CAD build for the part. Positions are in the model's coordinates, mm. A direction names the side the tool comes from. Give positions to 0.01 mm unless a question says otherwise; leave off trailing zeros. Order: outer loops, then holes, each group sorted by start corner. A loop starts at its lowest first (then second) coordinate and runs counter-clockwise, first axis right, second up.
Item 1: Wall check: L1, parallel to Y at x = 105, z = 1.8; L2, parallel to Y at x = 94.5, z = 2.8; L3, parallel to X at y = 18.5, z = 1.75. Give the ranges that are in metal, low to high.
Item 2: Flat gauge pin, fed straight in: P1, Ø2.5, axis at x = 10, y = 10, coming from the +Z side (3 decimals). Where does the tip first touch, or does it go through?
Item 3: Band-saw the part on A-A on y = 18. Give the cut face in (x, z).
Item 4: Two-plate mould, pull along X, no slides. Class faces 1 (the flat face through (56, 18, 0)), 2 (the cylindrical face through (10.761, 8.536, 1.479)), 3 (the flat face through (113, 18, 1)): released by +X, released by -X, zero draft, split by the parting line, or undercut.
Item 5: Band-saw the part on B-B on x = 18. Give the cut face in (y, z).
Item 6: Band-saw the part on D-D on x = 67.5. Give the cut face in (y, z).
Item 7: Which spindle directions (+Z, -Z, +X, -X, +Y, -Y) get a long thin tool onto all of the face, cutting with end or side? Do faces 4 (the cylindrical face through (0.57, 0.6, 1.52)), 5 (the cylindrical face through (24.35, 25.96, 1.48)). Say none if no direction does.
Item 8: Band-saw the part on C-C on z = 1.5. Count the separate pieces of the cut face and the enclosed holes in it, plus the area to 3 significant figures.
```python
from build123d import *

# Parameters (mm, degrees)
SKETCH_1_W      = 113
SKETCH_1_H      = 36
SKETCH_1_R      = 1.65
EXTRUDE_1_DEPTH = 3
FILLET_1_R      = 2


with BuildPart() as part:
    # 草图1 → 凸台-拉伸1 (new body)
    with BuildSketch(Plane.XY):
        with Locations((56.5, 18)):
            Rectangle(SKETCH_1_W, SKETCH_1_H)
        with Locations((10, 10)):
            Circle(SKETCH_1_R, mode=Mode.SUBTRACT)
        with Locations((18, 10)):
            Circle(SKETCH_1_R, mode=Mode.SUBTRACT)
        with BuildLine():
            ThreePointArc((26, 8.35), (24.35, 10), (26, 11.65))
            Line((26, 11.65), (97, 11.65))
            ThreePointArc((97, 11.65), (98.166726189, 11.166726189), (98.65, 10))
            ThreePointArc((98.65, 10), (98.166726189, 8.833273811), (97, 8.35))
            Line((97, 8.35), (26, 8.35))
        make_face(mode=Mode.SUBTRACT)
        with Locations((105, 10)):
            Circle(SKETCH_1_R, mode=Mode.SUBTRACT)
        with Locations((10, 18)):
            Circle(SKETCH_1_R, mode=Mode.SUBTRACT)
        with Locations((18, 18)):
            Circle(SKETCH_1_R, mode=Mode.SUBTRACT)
        with Locations((10, 26)):
            Circle(SKETCH_1_R, mode=Mode.SUBTRACT)
        with Locations((18, 26)):
            Circle(SKETCH_1_R, mode=Mode.SUBTRACT)
        with BuildLine():
            ThreePointArc((26, 24.35), (24.35, 26), (26, 27.65))
            Line((26, 27.65), (97, 27.65))
            ThreePointArc((97, 27.65), (98.166726189, 27.166726189), (98.65, 26))
            ThreePointArc((98.65, 26), (98.166726189, 24.833273811), (97, 24.35))
            Line((97, 24.35), (26, 24.35))
        make_face(mode=Mode.SUBTRACT)
        with Locations((97, 18)):
            Circle(SKETCH_1_R, mode=Mode.SUBTRACT)
        with Locations((105, 18)):
            Circle(SKETCH_1_R, mode=Mode.SUBTRACT)
        with Locations((105, 26)):
            Circle(SKETCH_1_R, mode=Mode.SUBTRACT)
    extrude(amount=EXTRUDE_1_DEPTH)

    # 圆角1
    fillet_1_edges = [part.edges().sort_by_distance(p)[0] for p in [
        (0, 0, 1.5),
        (0, 36, 1.5),
        (113, 36, 1.5),
        (113, 0, 1.5),
    ]]
    fillet(fillet_1_edges, radius=FILLET_1_R)


solid = part.part
```
The answers:
1. L1: y = 0 to 8.35, 11.65 to 16.35, 19.65 to 24.35, 27.65 to 36
1. L2: y = 0 to 8.35, 11.65 to 24.35, 27.65 to 36
1. L3: x = 0 to 8.43, 11.57 to 16.43, 19.57 to 95.43, 98.57 to 103.43, 106.57 to 113
2. P1: passes through
3. outline: (0, 0) - (8.35, 0) - (8.35, 3) - (0, 3) - close; (11.65, 0) - (16.35, 0) - (16.35, 3) - (11.65, 3) - close; (19.65, 0) - (95.35, 0) - (95.35, 3) - (19.65, 3) - close; (98.65, 0) - (103.35, 0) - (103.35, 3) - (98.65, 3) - close; (106.65, 0) - (113, 0) - (113, 3) - (106.65, 3) - close
4. face 1: zero draft
4. face 2: undercut
4. face 3: released by +X
5. outline: (0, 0) - (8.35, 0) - (8.35, 3) - (0, 3) - close; (11.65, 0) - (16.35, 0) - (16.35, 3) - (11.65, 3) - close; (19.65, 0) - (24.35, 0) - (24.35, 3) - (19.65, 3) - close; (27.65, 0) - (36, 0) - (36, 3) - (27.65, 3) - close
6. outline: (0, 0) - (8.35, 0) - (8.35, 3) - (0, 3) - close; (11.65, 0) - (24.35, 0) - (24.35, 3) - (11.65, 3) - close; (27.65, 0) - (36, 0) - (36, 3) - (27.65, 3) - close
7. face 4: +Z, -Z, -X, -Y
7. face 5: +Z, -Z
8. separate pieces: 1
8. enclosed holes: 12
8. area: 3,490 mm2
